```python
from build123d import *

# Parameters (mm, degrees)
CABBOTTOM_OUTLINE_W       = 1282.7
CABBOTTOM_OUTLINE_H       = 603.25
CABBOTTOM_THICKNESS_DEPTH = 17.78
SKETCH4_R                 = 22.225
SKETCH4_R_2               = 1.5875
SKETCH4_R_3               = 1.628860789
SKETCH4_R_4               = 1.721410862
CUT_EXTRUDE1_DEPTH        = 17.78
BRACECUTS_DEPTH_DEPTH     = 5.08


with BuildPart() as part:
    # CabBottom_Outline → CabBottom_Thickness (new body)
    with BuildSketch(Plane.XY):
        with Locations((9556.220833334, -6075.3625)):
            Rectangle(CABBOTTOM_OUTLINE_W, CABBOTTOM_OUTLINE_H)
    extrude(amount=-CABBOTTOM_THICKNESS_DEPTH)

    # Sketch4 → Cut-Extrude1 (cut)
    with BuildSketch(Plane.XY):
        with Locations((9051.395833334, -6316.6625)):
            Circle(SKETCH4_R)
        with Locations((9019.645833334, -6284.9125)):
            Circle(SKETCH4_R_2)
        with Locations((9083.145833334, -6284.9125)):
            Circle(SKETCH4_R_2)
        with Locations((9083.145833334, -6348.4125)):
            Circle(SKETCH4_R_3)
        with Locations((9019.645833334, -6348.4125)):
            Circle(SKETCH4_R_4)
        with Locations((9341.1675, -6265.8625)):
            Circle(SKETCH4_R_2)
        with Locations((9341.1675, -6138.8625)):
            Circle(SKETCH4_R_2)
        with Locations((9341.1675, -6011.8625)):
            Circle(SKETCH4_R_2)
        with Locations((9341.1675, -5884.8625)):
            Circle(SKETCH4_R_2)
        with Locations((9771.274166666, -5884.8625)):
            Circle(SKETCH4_R_2)
        with Locations((9771.274166666, -6011.8625)):
            Circle(SKETCH4_R_2)
        with Locations((9771.274166666, -6138.8625)):
            Circle(SKETCH4_R_2)
        with Locations((9771.274166666, -6265.8625)):
            Circle(SKETCH4_R_2)
        with BuildLine():
            Line((9974.787433334, -6061.075), (9974.787433334, -6045.241805286))
            ThreePointArc((9974.787433334, -6045.241805286), (9972.570596663, -6041.216758148), (9967.983861906, -6040.938848899))
            ThreePointArc((9967.983861906, -6040.938848899), (9957.371664972, -6048.421731638), (9949.888782233, -6059.033928571))
            ThreePointArc((9949.888782233, -6059.033928571), (9950.166691482, -6063.620663329), (9954.19173862, -6065.8375))
            Line((9954.19173862, -6065.8375), (9970.024933334, -6065.8375))
            ThreePointArc((9970.024933334, -6065.8375), (9973.39252938, -6064.442596045), (9974.787433334, -6061.075))
        make_face()
        with BuildLine():
            Line((9993.837433334, -6045.241805286), (9993.837433334, -6061.075))
            ThreePointArc((9993.837433334, -6061.075), (9995.232337289, -6064.442596045), (9998.599933334, -6065.8375))
            Line((9998.599933334, -6065.8375), (10014.433128046, -6065.8375))
            ThreePointArc((10014.433128046, -6065.8375), (10018.458175184, -6063.620663329), (10018.736084433, -6059.033928571))
            ThreePointArc((10018.736084433, -6059.033928571), (10011.253201696, -6048.421731637), (10000.641004763, -6040.938848899))
            ThreePointArc((10000.641004763, -6040.938848899), (9996.054270005, -6041.216758148), (9993.837433334, -6045.241805286))
        make_face()
        with BuildLine():
            Line((10014.433128046, -6084.8875), (9998.599933334, -6084.8875))
            ThreePointArc((9998.599933334, -6084.8875), (9995.232337289, -6086.282403955), (9993.837433334, -6089.65))
            Line((9993.837433334, -6089.65), (9993.837433334, -6105.483194714))
            ThreePointArc((9993.837433334, -6105.483194714), (9996.054270005, -6109.508241852), (10000.641004763, -6109.786151102))
            ThreePointArc((10000.641004763, -6109.786151102), (10011.253201699, -6102.303268365), (10018.736084435, -6091.691071429))
            ThreePointArc((10018.736084435, -6091.691071429), (10018.458175184, -6087.104336671), (10014.433128046, -6084.8875))
        make_face()
        with BuildLine():
            Line((9970.024933334, -6084.8875), (9954.19173862, -6084.8875))
            ThreePointArc((9954.19173862, -6084.8875), (9950.166691482, -6087.104336671), (9949.888782233, -6091.691071429))
            ThreePointArc((9949.888782233, -6091.691071429), (9957.371664972, -6102.303268362), (9967.983861906, -6109.786151101))
            ThreePointArc((9967.983861906, -6109.786151101), (9972.570596663, -6109.508241852), (9974.787433334, -6105.483194714))
            Line((9974.787433334, -6105.483194714), (9974.787433334, -6089.65))
            ThreePointArc((9974.787433334, -6089.65), (9973.39252938, -6086.282403955), (9970.024933334, -6084.8875))
        make_face()
        with BuildLine():
            ThreePointArc((9890.650044519, -6058.044318182), (9916.960512426, -6008.010579092), (9966.994251516, -5981.700111185))
            ThreePointArc((9966.994251516, -5981.700111185), (9972.584359078, -5978.426082773), (9974.787433334, -5972.333872304))
            ThreePointArc((9974.787433334, -5972.333872304), (9971.354643804, -5965.01194656), (9963.530615152, -5962.967633422))
            ThreePointArc((9963.530615152, -5962.967633422), (9903.490128244, -5994.54019491), (9871.917566756, -6054.580681818))
            ThreePointArc((9871.917566756, -6054.580681818), (9879.551987456, -6065.678738882), (9890.650044519, -6058.044318182))
        make_face()
        with BuildLine():
            ThreePointArc((9890.650044519, -6092.680681818), (9916.960512426, -6142.714420908), (9966.994251516, -6169.024888814))
            ThreePointArc((9966.994251516, -6169.024888814), (9974.628672216, -6180.122945878), (9963.530615152, -6187.757366578))
            ThreePointArc((9963.530615152, -6187.757366578), (9903.490128244, -6156.18480509), (9871.917566756, -6096.144318182))
            ThreePointArc((9871.917566756, -6096.144318182), (9879.551987456, -6085.046261119), (9890.650044519, -6092.680681818))
        make_face()
        with BuildLine():
            ThreePointArc((10001.630615152, -6169.024888815), (10051.664354242, -6142.714420908), (10077.974822149, -6092.680681818))
            ThreePointArc((10077.974822149, -6092.680681818), (10089.072879212, -6085.046261118), (10096.707299912, -6096.144318182))
            ThreePointArc((10096.707299912, -6096.144318182), (10065.134738424, -6156.18480509), (10005.094251516, -6187.757366578))
            ThreePointArc((10005.094251516, -6187.757366578), (9993.996194453, -6180.122945878), (10001.630615152, -6169.024888815))
        make_face()
        with BuildLine():
            ThreePointArc((10001.630615152, -5981.700111185), (10051.664354242, -6008.010579092), (10077.974822148, -6058.044318182))
            ThreePointArc((10077.974822148, -6058.044318182), (10089.072879212, -6065.678738882), (10096.707299912, -6054.580681818))
            ThreePointArc((10096.707299912, -6054.580681818), (10065.134738424, -5994.54019491), (10005.094251516, -5962.967633422))
            ThreePointArc((10005.094251516, -5962.967633422), (9993.996194453, -5970.602054122), (10001.630615152, -5981.700111185))
        make_face()
        with BuildLine():
            ThreePointArc((9917.282231904, -6111.603251872), (9908.112433335, -6075.3625), (9917.282231902, -6039.121748127))
            ThreePointArc((9917.282231902, -6039.121748127), (9930.191101067, -6035.273066932), (9934.039782262, -6048.181936096))
            ThreePointArc((9934.039782262, -6048.181936096), (9927.162433334, -6075.3625), (9934.039782262, -6102.543063904))
            ThreePointArc((9934.039782262, -6102.543063904), (9930.191101067, -6115.451933067), (9917.282231904, -6111.603251872))
        make_face()
        with BuildLine():
            ThreePointArc((9948.071681461, -6008.332298571), (9984.312433334, -5999.162499998), (10020.553185206, -6008.33229857))
            ThreePointArc((10020.553185206, -6008.33229857), (10024.4018664, -6021.241167734), (10011.492997237, -6025.089848928))
            ThreePointArc((10011.492997237, -6025.089848928), (9984.312433333, -6018.212500001), (9957.131869429, -6025.089848928))
            ThreePointArc((9957.131869429, -6025.089848928), (9944.223000266, -6021.241167734), (9948.071681461, -6008.332298571))
        make_face()
        with BuildLine():
            ThreePointArc((10020.553185206, -6142.39270143), (9984.312433334, -6151.5625), (9948.071681462, -6142.39270143))
            ThreePointArc((9948.071681462, -6142.39270143), (9944.223000267, -6129.483832267), (9957.13186943, -6125.635151072))
            ThreePointArc((9957.13186943, -6125.635151072), (9984.312433334, -6132.5125), (10011.492997238, -6125.635151072))
            ThreePointArc((10011.492997238, -6125.635151072), (10024.401866401, -6129.483832267), (10020.553185206, -6142.39270143))
        make_face()
        with BuildLine():
            ThreePointArc((10051.342634764, -6039.121748128), (10060.512433334, -6075.362500001), (10051.342634763, -6111.603251873))
            ThreePointArc((10051.342634763, -6111.603251873), (10038.43373034, -6115.45201683), (10034.585084407, -6102.543063904))
            ThreePointArc((10034.585084407, -6102.543063904), (10041.481320453, -6075.344350738), (10034.638263059, -6048.132209422))
            ThreePointArc((10034.638263059, -6048.132209422), (10038.489595862, -6035.282908491), (10051.342634764, -6039.121748128))
        make_face()
    extrude(amount=-CUT_EXTRUDE1_DEPTH, mode=Mode.SUBTRACT)

    # BraceCuts → BraceCuts_Depth (cut)
    with BuildSketch(Plane.XY):
        Polygon((9350.0575, -6075.3625), (9350.0575, -5773.7375), (9332.2775, -5773.7375), (9332.2775, -6376.9875), (9350.0575, -6376.9875), align=None)
        Polygon((9762.384166666, -6075.3625), (9762.384166666, -6376.9875), (9780.164166666, -6376.9875), (9780.164166666, -5773.7375), (9762.384166666, -5773.7375), align=None)
    extrude(amount=-BRACECUTS_DEPTH_DEPTH, mode=Mode.SUBTRACT)


solid = part.part
```
Build history of the part. All positions in model axes, mm. A direction names the side the tool comes from. Give positions to 0.01 mm unless a question says otherwise; leave off trailing zeros. One line per question, with ' | ' between items. Start each with the question number.
1) 3-axis set-ups, long thin cutter, end or side, ignore diameter. For faces 1 (the cylindrical face through (10065.814, -6155.5, -8.766)), 2 (the flat face through (9547, -6071, -17.78)): which of +Z, -Z, +X, -X, +Y, -Y reach the whole face in a straight line?
2) Probe L1, parallel to X at y = -6221, z = -3; L2, parallel to X at y = -5998, z = -16.5; L3, parallel to Y at x = 9053, z = -16.5. List the from-to ranges inside material, lowest first.
3) Cut at A-A (z = -8.25). Count the separate pieces of the cut face and the enclosed holes in it, plus the area to 3 significant figures.
4) Two-plate mould, pull along Y, no slides. Class faces 3 (the cylindrical face through (10051.094, -6143.28, -8.766)), 4 (the cylindrical face through (10065.81, -5995.22, -8.77)), 5 (the flat face through (9121, -6071, 0)): released by +Y, released by -Y, zero draft, split by the parting line, or undercut.
5) Pin check, flat tip, straight feed: pin 1 (9 mm diameter, centred on x = 9774.5, y = -6207.5, fed in from +Z). Stop position of the tip, or through.
Return value:
1) face 1: +Z, -Z | face 2: -Z, +X, -X, +Y, -Y
2) L1: 8914.87 to 9332.28, 9350.06 to 9762.38, 9780.16 to 10197.57 | L2: 8914.87 to 9900.17, 9928.75 to 10039.88, 10068.45 to 10197.57 | L3: -6376.99 to -6338.83, -6294.5 to -5773.74
3) separate pieces: 1 | enclosed holes: 25 | area: 753,000 mm^2
4) face 3: undercut | face 4: undercut | face 5: zero draft
5) pin 1: z = -5.08
